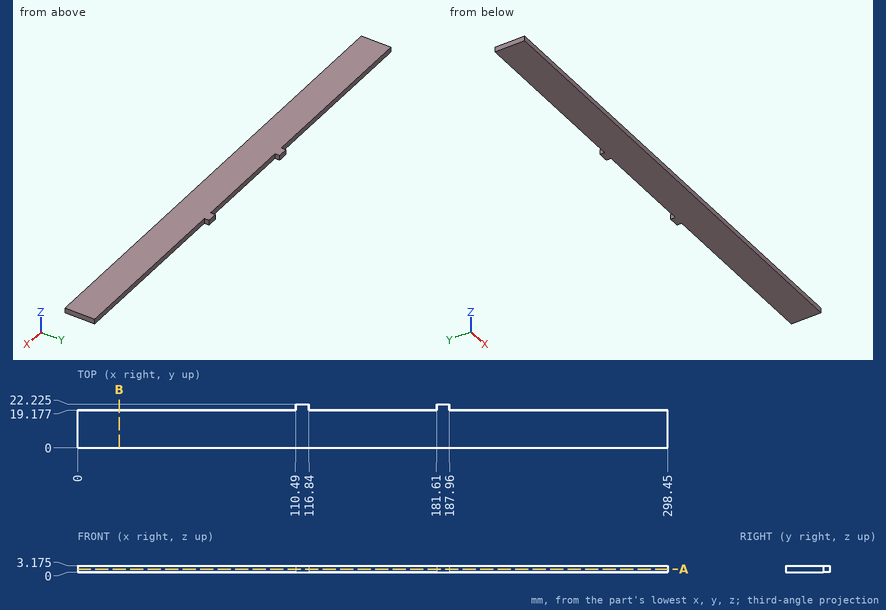
Print and shaded views of the part. All mm, measured from the part's lowest x, y and z. Coordinates: 2 decimals unless noted, no trailing zeros. Loops run counter-clockwise (first coordinate to the right, second up) from the corner with the lowest first, then second, coordinate; pieces in that order, holes last. Notation, with made-up numbers: (28.5, 53.25) -> (48.5, 53.25) arc R15 ccw to (48.5, 82.25) -> close; hole circle Ø6 at (20.5, 36). An arc over 180 degrees is marked (long way). Use one line per item in the form item = value. Start each with the question number.
(1) Flat gauge pins, fed straight in: pin 1 (0.9 mm diameter, centred on y = 20, z = 1.5, fed in from -X); pin 2 (1.6 mm diameter, centred on x = 240.5, z = 2, fed in from +Y); pin 3 (10 mm diameter, centred on x = 74, y = 8.5, fed in from -Z). Where does each tip first touch, or does it go through?
(2) Cut at A-A on z = 1.55. Give the cut face in (x, y) (3 decimals).
(3) Cut at B-B on x = 21. Give the cut face in (y, z) (3 decimals).
(4) Probe probe 1 along X at (y, z) = (20, 1.7); probe 2 along Y at (x, z) = (266, 2.25). List the from-to ranges inside material, lowest first. Write a range as from..to.
Values:
q1.pin_1 = 110.49
q1.pin_2 = 19.18
q1.pin_3 = 0
q2.outline = (0, 0) -> (298.45, 0) -> (298.45, 19.177) -> (187.96, 19.177) -> (187.96, 22.225) -> (181.61, 22.225) -> (181.61, 19.177) -> (116.84, 19.177) -> (116.84, 22.225) -> (110.49, 22.225) -> (110.49, 19.177) -> (0, 19.177) -> close
q3.outline = (0, 0) -> (19.177, 0) -> (19.177, 3.175) -> (0, 3.175) -> close
q4.probe_1 = 110.49..116.84, 181.61..187.96
q4.probe_2 = 0..19.18
